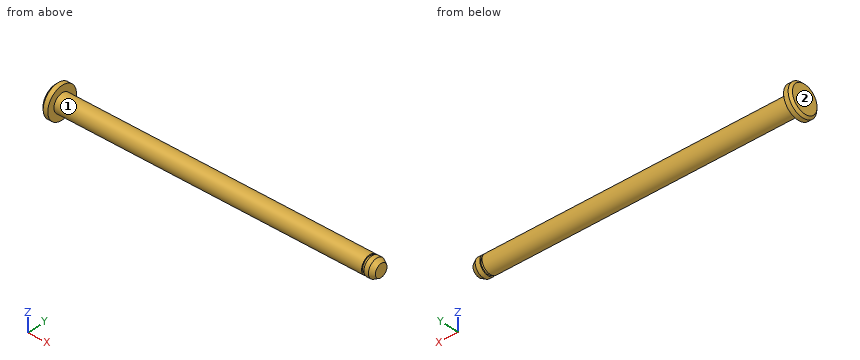
Autodesk Inventor part; units mm, degrees
ref_plane "YZ Plane" through (0, 0, 0) normal (1, 0, 0) x (0, 1, 0)
ref_plane "XZ Plane" through (0, 0, 0) normal (0, 1, 0) x (-1, 0, 0)
ref_plane "XY Plane" through (0, 0, 0) normal (0, 0, 1) x (1, 0, 0)
sketch "Szkic1" plane through (0, 0, 0) normal (0, 0, 1) x (1, 0, 0)
  line L0 (-3, 0) -> (-3, 7)
  line L1 (-3, 7) -> (0, 7)
  line L2 (0, 7) -> (0, 4)
  line L3 (0, 4) -> (140, 4)
  line L4 (140, 4) -> (140, 0)
  line L5 (-3, 0) -> (140, 0)
  line L6 (-31.6, 0) -> (168.6, 0)
  line L7 (0, -1.4) -> (0, 8.4)
  dimension "d0" = 3
  dimension "d1" = 140
  dimension "d2" = 8
  dimension "d3" = 14
revolve "Bryła" add sketch "Szkic1" angle 360 about axis through (-3, 0, 0) along (1, 0, 0)
chamfer "Faza1" distance 2 angle 30 1 edges at (140, -4, 0) measured on face at (46.6667, 3.987, -0.3219)
chamfer "Faza2" distance 1 angle 45 1 edges at (-3, -7, 0) measured on face at (-2, 6.9773, -0.5633)
ref_plane "Płaszczyzna konstrukcyjna1" through (135, 0, 0) normal (1, 0, 0) x (0, 0, -1)
sketch "Szkic2" plane through (135, 0, 0) normal (1, 0, 0) x (0, 0, -1)
  circle A0 centre (0, 0) radius 2.8453
  circle A1 centre (0, 0) radius 4
  circle A2 centre (0, 0) radius 4
  circle A3 centre (0, 0) radius 3.5
  point P0 (0, 0)
  dimension "d16" = 7
extrude "Wyciągnięcie proste1" cut sketch "Szkic2" along normal blind 1 contours A1
equation "\"d0\" = KOH"
equation "\"d2\" = NND"
equation "\"d3\" = KOD"
equation "\"d7\" = PHH1"
equation "\"d8\" = FAWI1"
equation "\"d12\" = PHH1"
equation "\"d4\" = PHH2"
equation "\"d6\" = FAWI2"
equation "\"d13\" = PHH2"
equation "\"KOH\" = 3"
equation "\"KOD\" = 14"
equation "\"NND\" = 8"
equation "\"FAWI1\" = 30deg"
equation "\"FAWI2\" = 45deg"
equation "\"PHH2\" = 1"
equation "\"PHH1\" = 2"
properties part number "ISO 2341 - A - 8 x 70" material "Stal"
Build history of the part. All positions in model axes, mm. Face numbers are marked on the shaded views. A direction names the side the tool comes from. Coordinates: 2 decimals unless noted, no trailing zeros. Write each loop counter-clockwise with the first axis right and the second up, starting at its lowest first coordinate (ties: lowest second). Pieces come first, ordered by that corner, then holes.
(1) Drill centre lines: line 1 (X direction, y = 1.75, z = 3.75); line 2 (X direction, y = 3.5, z = -0.5); line 3 (Z direction, x = 7, y = 0). Where is each one in solid material? Low to high.
(2) Cut at C-C on x = 54. List the corners of the cut face in (y, z), and give its area (3 significant figures).
(3) Cut at A-A on y = 0. List the corners of the cut face in (x, z), and give its area (3 significant figures).
(4) 3-axis set-ups, long thin cutter, end or side, ignore diameter. For the marked faces 1 and 2: which of +Z, -Z, +X, -X, +Y, -Y reach the whole face in a straight line?
(5) Pin check, flat tips, straight feed: pin 1 Ø8 at (x, z) = (79, 2.5) entering from +Y; pin 2 Ø4 at (x, y) = (94, 2.5) entering from +Z; pin 3 Ø1.5 at (x, y) = (116, 1) entering from -Z. Stop position of each tip, or through.
Working result:
1. line 1: x = -3 to 0
1. line 2: x = -3 to 135, 136 to 138.8
1. line 3: z = -4 to 4
2. outline: circle Ø8 at (0, 0)
2. area: 50.3 mm2
3. outline: (-3, -6) - (-2, -7) - (0, -7) - (0, -4) - (135, -4) - (135, -3.5) - (136, -3.5) - (136, -4) - (138, -4) - (140, -2.85) - (140, 2.85) - (138, 4) - (136, 4) - (136, 3.5) - (135, 3.5) - (135, 4) - (0, 4) - (0, 7) - (-2, 7) - (-3, 6) - close
3. area: 1,160 mm2
4. face 1: +X
4. face 2: +Z, -Z, -X, +Y, -Y
5. pin 1: stops at y = 4
5. pin 2: stops at z = 3.97
5. pin 3: stops at z = -3.99
